Input: part model. Units: mm. Frame: model coordinates. A direction names the side the tool comes from. Coordinates: 2 decimals unless noted, no trailing zeros. Order: outer loops, then holes, each group sorted by start corner. A loop starts at its lowest first (then second) coordinate and runs counter-clockwise, first axis right, second up.
from build123d import *

# Parameters (mm, degrees)
EXTRUDE_1_DEPTH     = 50
CUT_EXTRUDE_START   = -19.5
SKETCH_2_R          = 1.5
CUT_EXTRUDE_1_DEPTH = 70
SKETCH_3_OUTSIDE_W  = 61.218
SKETCH_3_OUTSIDE_H  = 66.218
CUT_EXTRUDE_2_DEPTH = 70
SKETCH_2_3_R        = 1.5
CUT_EXTRUDE_4_DEPTH = 10
SKETCH_5_R          = 1
CUT_EXTRUDE_5_DEPTH = 10
FILLET_1_R          = 5
SKETCH_6_W          = 13
SKETCH_6_H          = 23.5
CUT_EXTRUDE_6_DEPTH = 10
SKETCH_7_R          = 1.65
CUT_EXTRUDE_7_DEPTH = 10
SKETCH_8_W          = 14
SKETCH_8_H          = 14
CUT_EXTRUDE_8_DEPTH = 10


with BuildPart() as part:
    # 草图1 → 凸台-拉伸1 (new body)
    with BuildSketch(Plane.XY):
        Polygon((-45, 11.5), (0, 11.5), (0, -11.5), (-45, -11.5), (-45, -8), (-3.5, -8), (-3.5, 8), (-45, 8), align=None)
    extrude(amount=EXTRUDE_1_DEPTH)

    # 草图2 → 切除-拉伸1 (cut)
    with BuildSketch(Plane.XZ.offset(11.5).offset(CUT_EXTRUDE_START)):
        with Locations((-16, 35)):
            Circle(SKETCH_2_R)
        with Locations((-16, 15)):
            Circle(SKETCH_2_R)
        with Locations((-31, 30)):
            Circle(SKETCH_2_R)
        with Locations((-31, 20)):
            Circle(SKETCH_2_R)
    extrude(amount=-CUT_EXTRUDE_1_DEPTH, mode=Mode.SUBTRACT)

    # 草图3 outside → 切除-拉伸2 (cut)
    with BuildSketch(Plane.XZ.offset(11.5)):
        with Locations((-22.5, 25)):
            Rectangle(SKETCH_3_OUTSIDE_W, SKETCH_3_OUTSIDE_H)
        Polygon((-21, 0), (-36, 15), (-36, 35), (-21, 50), (0, 50), (0, 0), align=None, mode=Mode.SUBTRACT)
    extrude(amount=-CUT_EXTRUDE_2_DEPTH, mode=Mode.SUBTRACT)

    # 草图2<3> → 切除-拉伸4 (cut)
    with BuildSketch(Plane.XZ.offset(11.5)):
        with Locations((-31, 30)):
            Circle(SKETCH_2_3_R)
        with Locations((-31, 20)):
            Circle(SKETCH_2_3_R)
    extrude(amount=-CUT_EXTRUDE_4_DEPTH, mode=Mode.SUBTRACT)

    # 草图5 → 切除-拉伸5 (cut)
    with BuildSketch(Plane.XZ.offset(11.5)):
        with Locations((-16, 43.045)):
            Circle(SKETCH_5_R)
        with Locations((-16, 15.375)):
            Circle(SKETCH_5_R)
    extrude(amount=-CUT_EXTRUDE_5_DEPTH, mode=Mode.SUBTRACT)

    # 圆角1
    fillet_1_edges = [part.edges().sort_by_distance(p)[0] for p in [
        (-21, -9.75, 0),
        (-21, 9.75, 0),
        (-21, -9.75, 50),
        (-21, 9.75, 50),
        (-36, 9.75, 35),
        (-36, -9.75, 35),
        (-36, 9.75, 15),
        (-36, -9.75, 15),
    ]]
    fillet(fillet_1_edges, radius=FILLET_1_R)

    # 草图6 → 切除-拉伸6 (cut)
    with BuildSketch(Plane.XZ.offset(11.5)):
        with Locations((-16, 29.21)):
            Rectangle(SKETCH_6_W, SKETCH_6_H)
    extrude(amount=-CUT_EXTRUDE_6_DEPTH, mode=Mode.SUBTRACT)

    # 草图7 → 切除-拉伸7 (cut)
    with BuildSketch(Plane(origin=(0, 0, 0), x_dir=(0, 0, -1), z_dir=(1, 0, 0))):
        with Locations((-10, 4)):
            Circle(SKETCH_7_R)
        with Locations((-40, 4)):
            Circle(SKETCH_7_R)
        with Locations((-10, -4)):
            Circle(SKETCH_7_R)
        with Locations((-40, -4)):
            Circle(SKETCH_7_R)
    extrude(amount=-CUT_EXTRUDE_7_DEPTH, mode=Mode.SUBTRACT)

    # 草图8 → 切除-拉伸8 (cut)
    with BuildSketch(Plane(origin=(0, 11.5, 0), x_dir=(1, 0, 0), z_dir=(0, 1, 0))):
        with Locations((-16, -35)):
            Rectangle(SKETCH_8_W, SKETCH_8_H)
    extrude(amount=-CUT_EXTRUDE_8_DEPTH, mode=Mode.SUBTRACT)


solid = part.part
Item 1: Cut plane D-D on z = 10. Return loops of the section in (x, y).
Response values:
outline: (-31, -11.5) - (0, -11.5) - (0, -5.65) - (-3.5, -5.65) - (-3.5, -8) - (-31, -8) - close; (-31, 8) - (-3.5, 8) - (-3.5, 5.65) - (0, 5.65) - (0, 11.5) - (-31, 11.5) - close; (-3.5, -2.35) - (0, -2.35) - (0, 2.35) - (-3.5, 2.35) - close
Item 2: Access query for faces 4 (the face through (-16, -10, 17.46)), 5 (the face through (-23, 10, 35)), 6 (the face through (-16, -10, 40.96)), 7 (the face through (-20.82, -9.73, 49.63)). Directions: +Z, -Z, +X, -X, +Y, -Y. A direction counts if a zero-diameter tool reaches every point of the face in a straight line with its end or side. Return the directions, or none.
Response values:
face 4: -Y
face 5: +Y
face 6: +Y, -Y
face 7: +Z, -X, +Y, -Y
Item 3: Cut plane C-C on x = -16. Return loops of the section in (y, z) (3 decimals), then the cut area to 3 significant figures.
Response values:
outline: (-11.5, 0) - (-8, 0) - (-8, 14.375) - (-11.5, 14.375) - close; (-11.5, 16.375) - (-8, 16.375) - (-8, 17.46) - (-11.5, 17.46) - close; (-11.5, 40.96) - (-8, 40.96) - (-8, 42.045) - (-11.5, 42.045) - close; (-11.5, 44.045) - (-8, 44.045) - (-8, 50) - (-11.5, 50) - close; (8, 0) - (11.5, 0) - (11.5, 13.5) - (8, 13.5) - close; (8, 16.5) - (11.5, 16.5) - (11.5, 28) - (8, 28) - close; (8, 42) - (11.5, 42) - (11.5, 50) - (8, 50) - close
area: 194 mm2
Item 4: Ray query, probe 1 along Y at (x, z) = (-1.35, 40); probe 2 along Z at (x, y) = (-16, -9.9) (3 decimals); probe 3 along Z at (x, y) = (-18, -9.75). Return the intervals inside material, ascending.
Response values:
probe 1: y = -11.5 to -5.65, -2.35 to 2.35, 5.65 to 11.5
probe 2: z = 0 to 14.375, 16.375 to 17.46, 40.96 to 42.045, 44.045 to 50
probe 3: z = 0 to 17.46, 40.96 to 50
Item 5: Cut plane A-A on y = 4. Return loops of the section in (x, z).
Response values:
outline: (-3.5, 0) - (0, 0) - (0, 8.35) - (-3.5, 8.35) - close; (-3.5, 11.65) - (0, 11.65) - (0, 38.35) - (-3.5, 38.35) - close; (-3.5, 41.65) - (0, 41.65) - (0, 50) - (-3.5, 50) - close
Item 6: Pin query (flat end, axial travel): pin 1 Ø10 at (x, y) = (-30, -2.5) entering from -Z (3 decimals); pin 2 Ø8 at (y, z) = (3.5, 31.5) entering from -X; pin 3 Ø2.5 at (x, z) = (-16, 15) entering from +Y; pin 4 Ø1.8 at (x, z) = (-16, 43.045) entering from -Y. Return the tip coordinate at first contact, or that it passes through.
Response values:
pin 1: passes through
pin 2: stops at x = -3.5
pin 3: stops at y = -8
pin 4: stops at y = 8
Item 7: Draft query along Y for faces 1 (the face through (-24, -8, 25)), 2 (the face through (-1.726, 3.368, 8.476)), 3 (the face through (-32.11, 9.73, 21.01)). Return one class per face: pulls with the +Y half, pulls with the -Y half, needs draft (parallel to the pull), parting line crosses it, or undercut.
Response values:
face 1: undercut
face 2: undercut
face 3: needs draft
Item 8: Cut plane B-B on z = 26.5. Return loops of the section in (x, y), then the cut area to 4 significant figures.
Response values:
outline: (-36, -11.5) - (-22.5, -11.5) - (-22.5, -8) - (-36, -8) - close; (-36, 8) - (-3.5, 8) - (-3.5, -8) - (-9.5, -8) - (-9.5, -11.5) - (0, -11.5) - (0, 11.5) - (-36, 11.5) - close
area: 262.5 mm2
